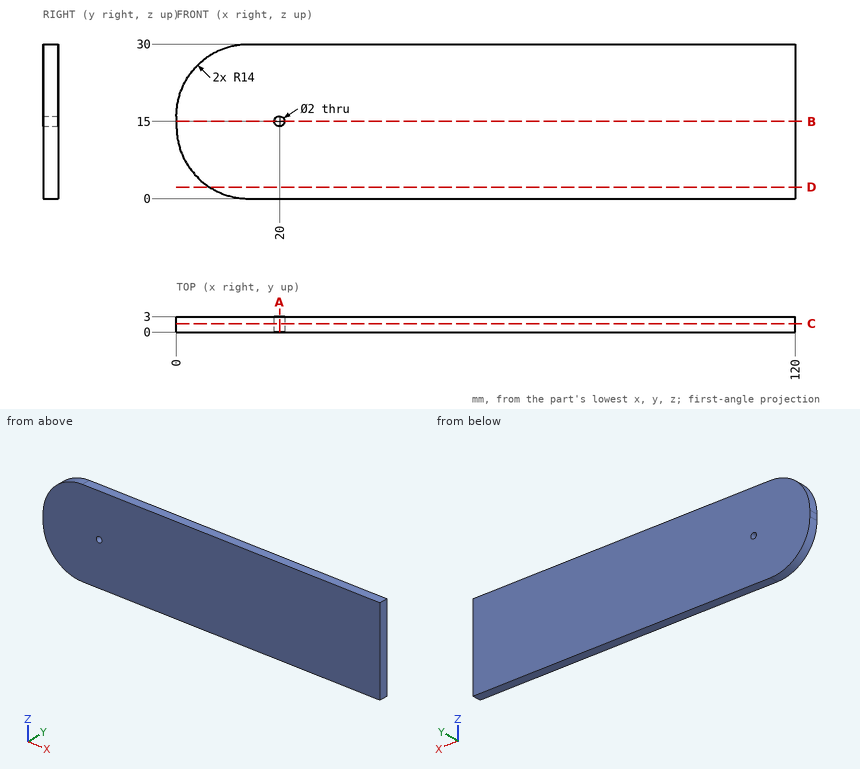
Study the drawing (mm; zero at the part's minimum x, y, z) and answer. Round coordinates to 2 decimals unless told otherwise and drop trailing zeros. Loops run counter-clockwise (first coordinate to the right, second up) from the corner with the lowest first, then second, coordinate; pieces in that order, holes last.
Q1. Section C-C, the plane y = 1.65 is taken. Determine the outline of the cut face in (x, z), then the cut area to 3 significant figures.
Q2. Section D-D, the plane z = 2.25 is taken. Determine the outline of the cut face in (x, y).
Q3. Find the intervals of material crossed by line 1 (X direction, y = 1.15, z = 15); line 2 (Z direction, x = 20, y = 2.35); line 3 (X direction, y = 1.3, z = 27.75), in increasing order.
Q4. Section A-A, the plane x = 20 is taken. Determine the outline of the cut face in (y, z).
Q5. Section B-B, the plane z = 15 is taken. Determine the outline of the cut face in (x, y).
Q6. Given pin 1 Ø2 at (x, z) = (34.5, 22) entering from -Y; pin 2 Ø1.6 at (x, z) = (20, 15) entering from +Y, each flat-ended and moving along its own axis, determine where each tip first touches the part or whether it passes through.
Completed:
1. outline: (0, 14) arc R14 ccw to (14, 0) - (120, 0) - (120, 30) - (14, 30) arc R14 ccw to (0, 16) - close; hole circle Ø2 at (20, 15)
1. area: 3,510 mm2
2. outline: (6.39, 0) - (120, 0) - (120, 3) - (6.39, 3) - close
3. line 1: x = 0 to 19, 21 to 120
3. line 2: z = 0 to 14, 16 to 30
3. line 3: x = 6.39 to 120
4. outline: (0, 0) - (3, 0) - (3, 14) - (0, 14) - close; (0, 16) - (3, 16) - (3, 30) - (0, 30) - close
5. outline: (0, 0) - (19, 0) - (19, 3) - (0, 3) - close; (21, 0) - (120, 0) - (120, 3) - (21, 3) - close
6. pin 1: stops at y = 0
6. pin 2: passes through
